Work out the finished part from the listing and answer in its coordinate system (mm). A direction names the side the tool comes from. Coordinates: 2 decimals unless noted, no trailing zeros. Write each question's results on one line, items separated by ' | '. Start each with the question number.
1. Determine the mould class of faces 1 (the flat face through (-5.2, 0, 3)), 2 (the flat face through (9, 15, 3)), 3 (the flat face through (-15, 9, 3)), 4 (the flat face through (5.2, 0, 3)) for opening direction Y: released by +Y, released by -Y, zero draft, split by the parting line, or undercut.
2. A cutting plane is placed at A-A on z = 141.5. State how many separate pieces and enclosed holes the cut face has, then the cut area to 3 significant figures.
3. Which of the six approach directions +Z, -Z, +X, -X, +Y, -Y give full straight-line access (tool end or side, diameter ignored) to faces 5 (the flat face through (0, -5.2, 3)), 6 (the flat face through (15, 9, 3))?
4. Find the intervals of material crossed by line 1 along Y through (x, z) = (-11, 99.5); line 2 along Y through (x, z) = (0, 0), in increasing order. Write a range as [from, to].
5. Each of these flat-tipped pins is pushed along its axis until it touches: P1, Ø2, axis at y = -1, z = -8, coming from the -X side; P2, Ø1, axis at x = 3, z = 151.5, coming from the -Y side; P3, Ø4, axis at y = 0, z = 194.5, coming from the +X side. Where does it stop, or does it pass through?
from build123d import *

# Parameters (mm, degrees)
SKETCH_R  = 2.5
PAD_DEPTH = 245


with BuildPart() as part:
    # Sketch → Pad (new body, symmetric)
    with BuildSketch(Plane.XY):
        with BuildLine():
            Line((14, 3.15), (12.2, 3.15))
            Line((12.2, 3.15), (12.2, 8.15))
            Line((12.2, 8.15), (9.634924, 8.15))
            Line((9.634924, 8.15), (5.2, 3.715076))
            Line((5.2, 3.715076), (5.2, -3.715076))
            Line((5.2, -3.715076), (9.634924, -8.15))
            Line((9.634924, -8.15), (12.2, -8.15))
            Line((12.2, -8.15), (12.2, -3.15))
            Line((12.2, -3.15), (14, -3.15))
            ThreePointArc((15, -4.15), (14.707107, -3.442893), (14, -3.15))
            Line((15, -4.15), (15, -13))
            ThreePointArc((13, -15), (14.414214, -14.414214), (15, -13))
            Line((13, -15), (4.15, -15))
            ThreePointArc((3.15, -14), (3.442893, -14.707107), (4.15, -15))
            Line((3.15, -14), (3.15, -12.2))
            Line((3.15, -12.2), (8.15, -12.2))
            Line((8.15, -12.2), (8.15, -9.634924))
            Line((8.15, -9.634924), (3.715076, -5.2))
            Line((3.715076, -5.2), (-3.715076, -5.2))
            Line((-3.715076, -5.2), (-8.15, -9.634924))
            Line((-8.15, -9.634924), (-8.15, -12.2))
            Line((-8.15, -12.2), (-3.15, -12.2))
            Line((-3.15, -12.2), (-3.15, -14))
            ThreePointArc((-4.15, -15), (-3.442893, -14.707107), (-3.15, -14))
            Line((-4.15, -15), (-13, -15))
            ThreePointArc((-15, -13), (-14.414214, -14.414214), (-13, -15))
            Line((-15, -4.15), (-15, -13))
            ThreePointArc((-14, -3.15), (-14.707107, -3.442893), (-15, -4.15))
            Line((-12.2, -3.15), (-14, -3.15))
            Line((-12.2, -8.15), (-12.2, -3.15))
            Line((-12.2, -8.15), (-9.634924, -8.15))
            Line((-5.2, -3.715076), (-9.634924, -8.15))
            Line((-5.2, 3.715076), (-5.2, -3.715076))
            Line((-9.634924, 8.15), (-5.2, 3.715076))
            Line((-12.2, 8.15), (-9.634924, 8.15))
            Line((-12.2, 3.15), (-12.2, 8.15))
            Line((-14, 3.15), (-12.2, 3.15))
            ThreePointArc((-15, 4.15), (-14.707107, 3.442893), (-14, 3.15))
            Line((-15, 13), (-15, 4.15))
            ThreePointArc((-13, 15), (-14.414214, 14.414214), (-15, 13))
            Line((-4.15, 15), (-13, 15))
            ThreePointArc((-3.15, 14), (-3.442893, 14.707107), (-4.15, 15))
            Line((-3.15, 12.2), (-3.15, 14))
            Line((-8.15, 12.2), (-3.15, 12.2))
            Line((-8.15, 9.634924), (-8.15, 12.2))
            Line((-3.715076, 5.2), (-8.15, 9.634924))
            Line((3.715076, 5.2), (-3.715076, 5.2))
            Line((8.15, 9.634924), (3.715076, 5.2))
            Line((8.15, 12.2), (8.15, 9.634924))
            Line((3.15, 12.2), (8.15, 12.2))
            Line((3.15, 14), (3.15, 12.2))
            ThreePointArc((4.15, 15), (3.442893, 14.707107), (3.15, 14))
            Line((13, 15), (4.15, 15))
            ThreePointArc((15, 13), (14.414214, 14.414214), (13, 15))
            Line((15, 4.15), (15, 13))
            ThreePointArc((14, 3.15), (14.707107, 3.442893), (15, 4.15))
        make_face()
        Circle(SKETCH_R, mode=Mode.SUBTRACT)
        with BuildLine():
            Line((9.2, 12.2), (11.2, 12.2))
            ThreePointArc((12.2, 11.2), (11.907107, 11.907107), (11.2, 12.2))
            Line((12.2, 11.2), (12.2, 9.2))
            Line((12.2, 9.2), (9.2, 9.2))
            Line((9.2, 9.2), (9.2, 12.2))
        make_face(mode=Mode.SUBTRACT)
        with BuildLine():
            ThreePointArc((-11.2, 12.2), (-11.907107, 11.907107), (-12.2, 11.2))
            Line((-12.2, 9.2), (-12.2, 11.2))
            Line((-9.2, 9.2), (-12.2, 9.2))
            Line((-9.2, 12.2), (-9.2, 9.2))
            Line((-11.2, 12.2), (-9.2, 12.2))
        make_face(mode=Mode.SUBTRACT)
        with BuildLine():
            ThreePointArc((-12.2, -11.2), (-11.907107, -11.907107), (-11.2, -12.2))
            Line((-9.2, -12.2), (-11.2, -12.2))
            Line((-9.2, -9.2), (-9.2, -12.2))
            Line((-12.2, -9.2), (-9.2, -9.2))
            Line((-12.2, -11.2), (-12.2, -9.2))
        make_face(mode=Mode.SUBTRACT)
        with BuildLine():
            ThreePointArc((11.2, -12.2), (11.907107, -11.907107), (12.2, -11.2))
            Line((12.2, -11.2), (12.2, -9.2))
            Line((12.2, -9.2), (9.2, -9.2))
            Line((9.2, -9.2), (9.2, -12.2))
            Line((9.2, -12.2), (11.2, -12.2))
        make_face(mode=Mode.SUBTRACT)
    extrude(amount=PAD_DEPTH, both=True)


solid = part.part
Values:
1) face 1: undercut | face 2: released by +Y | face 3: zero draft | face 4: undercut
2) separate pieces: 1 | enclosed holes: 5 | area: 392 mm^2
3) face 5: +Z, -Z | face 6: +Z, -Z, +X, +Y, -Y
4) line 1: [-15, -12.2], [-9.2, -8.15], [8.15, 9.2], [12.2, 15] | line 2: [-5.2, -2.5], [2.5, 5.2]
5) P1: x = -5.2 | P2: y = -14.76 | P3: x = 5.2
